Source: CAD feature listing. Evaluate the final solid. Frame: model axes, mm. A direction names the side the tool comes from. Give positions to 0.01 mm unless a question says otherwise; leave off trailing zeros. Write each loop counter-clockwise with the first axis right and the second up, starting at its lowest first coordinate (ties: lowest second). Pieces come first, ordered by that corner, then holes. Notation, with made-up numbers: (-28, 47.25) - (-8, 47.25) arc R26 ccw to (-8, 68.25) - close; hole circle Ø11 at (-14.5, 53). An arc over 180 degrees is marked (long way). Answer as a JSON object with one key per item and string values. Group by question number.
from build123d import *

# Parameters (mm, degrees)
IZIM1_W                     = 20
IZIM1_H                     = 33
IZIM1_R                     = 3.25
Y_KSEKLIK_EKSTR_ZYON1_DEPTH = 4
IZIM2_W                     = 20
IZIM2_H                     = 4
Y_KSEKLIK_EKSTR_ZYON2_DEPTH = 15
IZIM3_R                     = 1.75
KES_EKSTR_ZYON1_DEPTH       = 15


with BuildPart() as part:
    # Çizim1 → Yükseklik-Ekstrüzyon1 (new body)
    with BuildSketch(Plane.XY):
        with Locations((10, 16.5)):
            Rectangle(IZIM1_W, IZIM1_H)
        with Locations((10, 13.5)):
            Circle(IZIM1_R, mode=Mode.SUBTRACT)
    extrude(amount=Y_KSEKLIK_EKSTR_ZYON1_DEPTH)

    # Çizim2 → Yükseklik-Ekstrüzyon2 (add)
    with BuildSketch(Plane.XY.offset(4)):
        with Locations((10, 31)):
            Rectangle(IZIM2_W, IZIM2_H)
    extrude(amount=Y_KSEKLIK_EKSTR_ZYON2_DEPTH)

    # Çizim3 → Kes-Ekstrüzyon1 (cut)
    with BuildSketch(Plane(origin=(0, 33, 0), x_dir=(1, 0, 0), z_dir=(0, 1, 0))):
        with Locations(Location((10, -12, 0), (0, 0, 270))):
            Circle(IZIM3_R)
    extrude(amount=-KES_EKSTR_ZYON1_DEPTH, mode=Mode.SUBTRACT)


solid = part.part
Q1. Ray query, probe 1 along X at (y, z) = (31.05, 12); probe 2 along Z at (x, y) = (4.25, 20); probe 3 along Y at (x, z) = (3.75, 15.5). Return the intervals inside material, ascending. Write a range as [from, to].
Q2. Draft query along X for faces 1 (the cylindrical face through (6.753, 13.643, 1.972)), 2 (the cylindrical face through (11.5, 31, 12.9)), 3 (the flat face through (0, 18.9, 3.8)), 4 (the flat face through (10, 33, 9)). Return one class per face: released by +X, released by -X, zero draft, split by the parting line, or undercut.
Q3. Section A-A on z = 12. Return the cut outline in (x, y).
Q4. Reachability of faces 5 (the flat face through (10, 31, 19)), 6 (the flat face through (10, 29, 10)) from +Z, -Z, +X, -X, +Y, -Y: full face, straight path, thin tool, end or side. Return the list, or none.
Q5. Section C-C on y = 13.5. Return the cut outline in (x, z).
Q6. First-contact query: pin 1 Ø5 at (x, y) = (10, 13.5) entering from -Z; pin 2 Ø10 at (x, z) = (18, 15) entering from -Y; pin 3 Ø6 at (x, y) = (9, 9.5) entering from +Z. Flat tips, straight axial feed; report the tip coordinate or a pass-through.
Q7. Section B-B on x = 10. Return the cut outline in (y, z), then the cut area to 3 significant figures.
Q8. Section D-D on x = 7.5. Return the cut outline in (y, z), then the cut area to 3 significant figures.
Taken from the geometry:
{
 "1": {"probe 1": "x = [0, 8.25], [11.75, 20]", "probe 2": "z = [0, 4]", "probe 3": "y = [29, 33]"},
 "2": {"face 1": "undercut", "face 2": "undercut", "face 3": "released by -X", "face 4": "zero draft"},
 "3": {"outline": "(0, 29) - (8.25, 29) - (8.25, 33) - (0, 33) - close; (11.75, 29) - (20, 29) - (20, 33) - (11.75, 33) - close"},
 "4": {"face 5": "+Z, +X, -X, +Y, -Y", "face 6": "+Z, +X, -X, -Y"},
 "5": {"outline": "(0, 0) - (6.75, 0) - (6.75, 4) - (0, 4) - close; (13.25, 0) - (20, 0) - (20, 4) - (13.25, 4) - close"},
 "6": {"pin 1": "passes through", "pin 2": "stops at y = 29", "pin 3": "stops at z = 4"},
 "7": {"outline": "(0, 0) - (10.25, 0) - (10.25, 4) - (0, 4) - close; (16.75, 0) - (33, 0) - (33, 10.25) - (29, 10.25) - (29, 4) - (16.75, 4) - close; (29, 13.75) - (33, 13.75) - (33, 19) - (29, 19) - close", "area": "152 mm²"},
 "8": {"outline": "(0, 0) - (11.42, 0) - (11.42, 4) - (0, 4) - close; (15.58, 0) - (33, 0) - (33, 19) - (29, 19) - (29, 4) - (15.58, 4) - close", "area": "175 mm²"}
}
